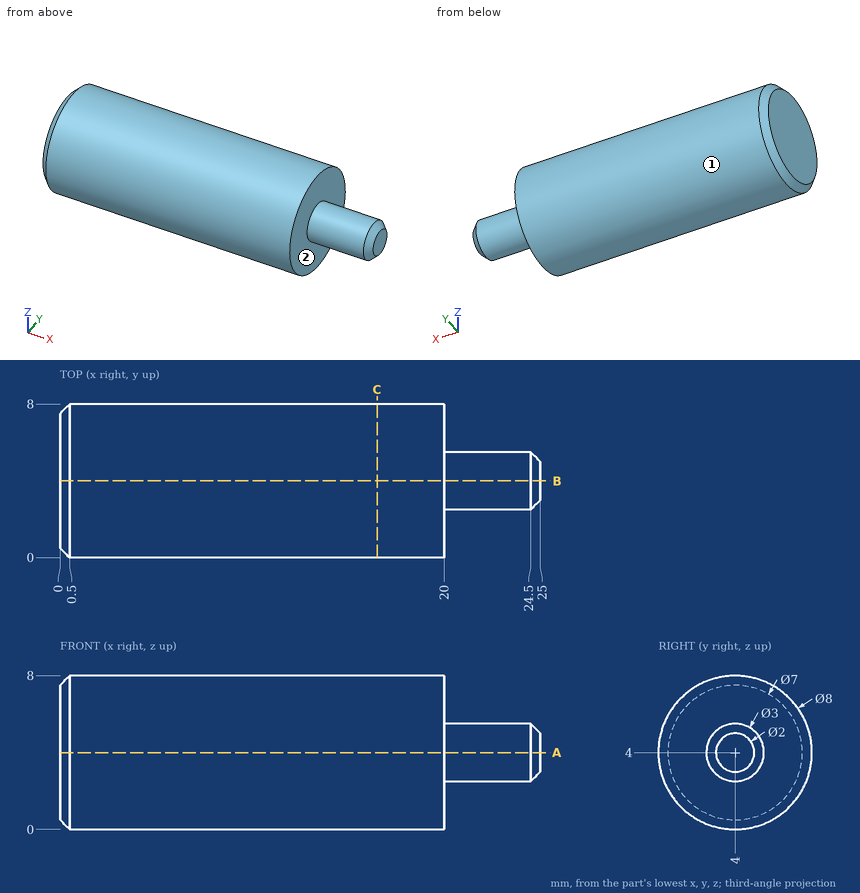
Can you work these out from the drawing? Everything is in mm from the part's minimum corner. A direction names the side the tool comes from. Round coordinates to 2 decimals unless told otherwise and drop trailing zeros. Write each loop counter-clockwise with the first axis right and the second up, starting at its lowest first coordinate (ties: lowest second). Pieces come first, ordered by that corner, then holes. Notation, with made-up numbers: (25, 18) - (66, 18) arc R22 cw to (66, 35) - close; hole circle Ø3 at (83.5, 15.25). An arc over 180 degrees is marked (long way). Write each question's results on one line, items separated by ' | '. Start each with the question number.
1) Which directions (+Z, -Z, +X, -X, +Y, -Y) give clear straight access to the entire face, cutting with the end or side of a thin tool? Please do the marked faces 1 and 2.
2) Suppose I cut it at C-C (x = 16.5). List the corners of the cut face in (y, z) for me, and give its area (3 significant figures).
3) Suppose I cut it at A-A (z = 4). List the corners of the cut face in (x, y) for me, and give its area (4 significant figures).
4) Please list where these lines run through material, in increasing order: line 1 (X direction, y = 4.5, z = 6.75); line 2 (X direction, y = 1, z = 2); line 3 (Y direction, x = 14.25, z = 2.75).
Here are the results:
1) face 1: +X, -X | face 2: +X
2) outline: circle Ø8 at (4, 4) | area: 50.3 mm2
3) outline: (0, 0.5) - (0.5, 0) - (20, 0) - (20, 2.5) - (24.5, 2.5) - (25, 3) - (25, 5) - (24.5, 5.5) - (20, 5.5) - (20, 8) - (0.5, 8) - (0, 7.5) - close | area: 174.5 mm2
4) line 1: x = 0 to 20 | line 2: x = 0.11 to 20 | line 3: y = 0.2 to 7.8
